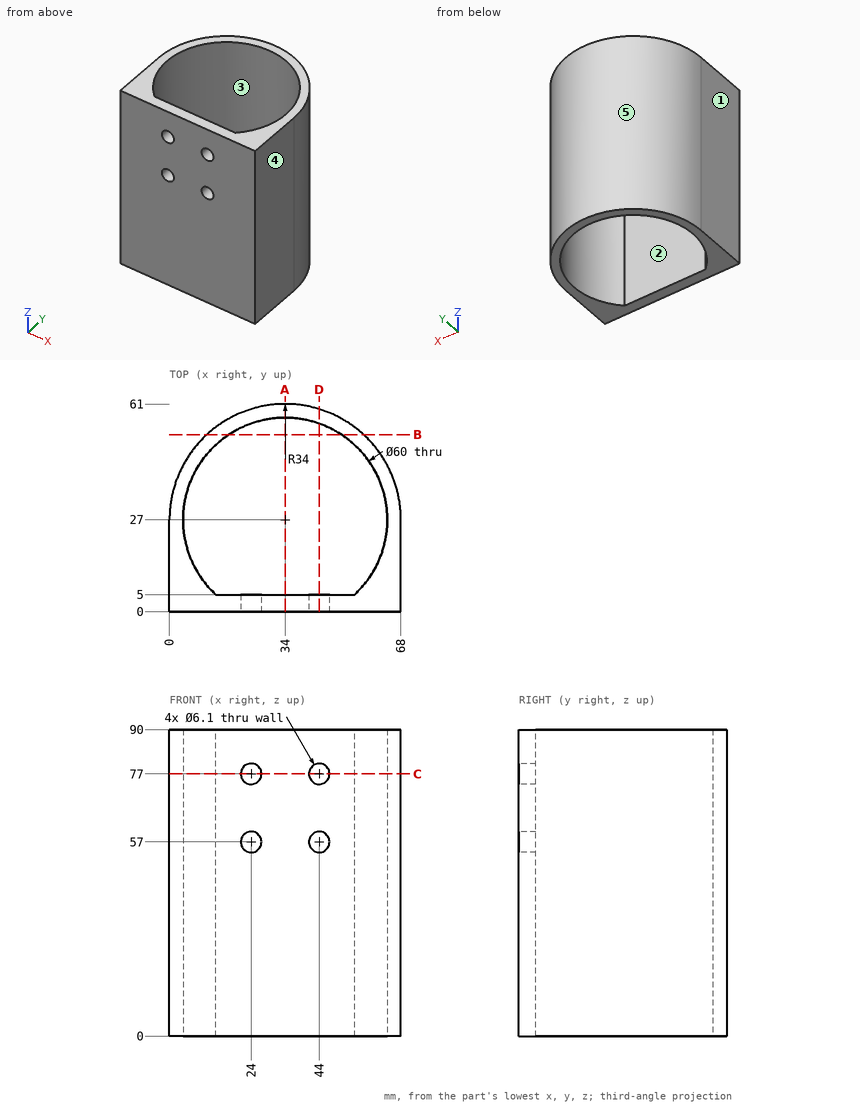
Geometry: see drawing. Coordinates: mm, zero at the bounding-box minimum. A direction names the side the tool comes from. Coordinates: 2 decimals unless noted, no trailing zeros. Loops run counter-clockwise (first coordinate to the right, second up) from the corner with the lowest first, then second, coordinate; pieces in that order, holes last. Notation, with made-up numbers: M -39,61 L -16,61 A27 ccw -16,98 Z; hole C -3.75,-7.75 d8. An arc over 180 degrees is marked long. Answer in a Markdown table with one row per item.
1. First-contact query: pin 1 (8 mm diameter, centred on x = 43, z = 70.5, fed in from +Y); pin 2 (2 mm diameter, centred on x = 21.5, z = 64.5, fed in from +Y); pin 3 (7 mm diameter, centred on x = 24, z = 77, fed in from +Y). Flat tips, straight axial feed; report the tip coordinate or a pass-through.
Response:
| item | result |
|---|---|
| pin 1 | stops at y = 60.63 |
| pin 2 | stops at y = 59 |
| pin 3 | stops at y = 60.37 |
2. Section A-A, the plane x = 34. Output: boundary loops of the cut face in (y, z), then the cut area to 3 significant figures.
Response:
| item | result |
|---|---|
| outline | M 0,0 L 5,0 L 5,90 L 0,90 Z; M 57,0 L 61,0 L 61,90 L 57,90 Z |
| area | 810 mm2 |
3. Section C-C, the plane z = 77. Output: boundary loops of the cut face in (x, y).
Response:
| item | result |
|---|---|
| outline | M 0,0 L 20.95,0 L 20.95,5 L 13.6,5 A30 cw long 54.4,5 L 47.05,5 L 47.05,0 L 68,0 L 68,27 A34 ccw 0,27 Z; M 27.05,0 L 40.95,0 L 40.95,5 L 27.05,5 Z |
4. Draft query along X for the marked faces 3, 4 and 5. Return one class per face: pulls with the +X half, pulls with the -X half, needs draft (parallel to the pull), parting line crosses it, or undercut.
Response:
| item | result |
|---|---|
| face 3 | undercut |
| face 4 | pulls with the +X half |
| face 5 | parting line crosses it |
5. Section D-D, the plane x = 44. Output: boundary loops of the cut face in (y, z), then the cut area to 3 significant figures.
Response:
| item | result |
|---|---|
| outline | M 0,0 L 5,0 L 5,53.95 L 0,53.95 Z; M 0,60.05 L 5,60.05 L 5,73.95 L 0,73.95 Z; M 0,80.05 L 5,80.05 L 5,90 L 0,90 Z; M 55.28,0 L 59.5,0 L 59.5,90 L 55.28,90 Z |
| area | 768 mm2 |
6. Reachability of the marked faces 1 and 2 from +Z, -Z, +X, -X, +Y, -Y: full face, straight path, thin tool, end or side. Return the list, or none.
Response:
| item | result |
|---|---|
| face 1 | +Z, -Z, -X, +Y, -Y |
| face 2 | +Z, -Z |
7. Section B-B, the plane y = 52. Output: boundary loops of the cut face in (x, z).
Response:
| item | result |
|---|---|
| outline | M 10.96,0 L 17.42,0 L 17.42,90 L 10.96,90 Z; M 50.58,0 L 57.04,0 L 57.04,90 L 50.58,90 Z |
8. Material intervals for line 1 (Z direction, x = 44, y = 2); line 2 (X direction, y = 27, z = 51); line 3 (Y direction, x = 34, z = 28), sorted ascending.
Response:
| item | result |
|---|---|
| line 1 | z = 0 to 53.95, 60.05 to 73.95, 80.05 to 90 |
| line 2 | x = 0 to 4, 64 to 68 |
| line 3 | y = 0 to 5, 57 to 61 |
